Here's how the part is built. I have some questions about the finished solid (model axes, mm). A direction names the side the tool comes from. Coordinates: 2 decimals unless noted, no trailing zeros. Write each loop counter-clockwise with the first axis right and the second up, starting at its lowest first coordinate (ties: lowest second). Pieces come first, ordered by that corner, then holes.
(1) For pin 1 Ø5 at (x, y) = (5.75, -5.75) entering from -Z; pin 2 Ø4 at (x, y) = (-5.75, 5.75) entering from +Z, each with a flat end and sliding along its axis, tell me the tip position at first contact or that it passes through.
(2) Please list where these lines run through material, in increasing order: probe 1 along X at (y, z) = (5.75, 12.75); probe 2 along X at (y, z) = (-0.25, 14); probe 3 along X at (y, z) = (-5.75, 11.75).
(3) Which directions (+Z, -Z, +X, -X, +Y, -Y) give clear straight access to the entire face, cutting with the end or side of a thin tool? Please do faces 4 (the cylindrical face through (8.8, -2.36, 7.693)), 5 (the cylindrical face through (-14.292, 10.035, 11.352)), 6 (the cylindrical face through (6.49, 4.33, 9.68)), 7 (the flat face through (-8.7, 6, 2)), 8 (the cylindrical face through (5.97, 9.36, 17.29)).
(4) Imagine slicing it at A-A, the plane z = 10. List the corners of the cut face in (x, y) for me, plus the area to 3 significant figures.
(5) Imagine slicing it at C-C, the plane x = 0. List the corners of the cut face in (y, z) for me, plus the area to 3 significant figures.
(6) Imagine slicing it at D-D, the plane y = 1.25. List the corners of the cut face in (x, z) for me.
(7) Thinking about a two-plate mould opening in Z: for faces 1 (the cylindrical face through (-6.1, -7.31, 9.68)), 2 (the cylindrical face through (5.708, 10.035, 11.352)), 3 (the flat face through (6, 4, 5)), which applies, released by +Z, released by -Z, zero draft, split by the parting line, or undercut?
```python
from build123d import *

# Parameters (mm, degrees)
F0_W      = 40
F0_H      = 25
F0_R      = 1.6
F0_R_2    = 5.1
F1_DEPTH  = 20
F2_R      = 5
F3_R      = 11.1
F4_DEPTH  = 5.5
F5_R      = 1.6
F6_DEPTH  = 5
F7_R      = 2.6
F8_DEPTH  = 25.001
F9_R      = 4.5
F9_R_2    = 2.6
F10_DEPTH = 5


with BuildPart() as f1:
    # F0 (on Top) → F1 (new body)
    with BuildSketch(Plane.XY):
        Rectangle(F0_W, F0_H)
        with Locations((-5.75, -5.75)):
            Circle(F0_R, mode=Mode.SUBTRACT)
        with Locations((5.75, -5.75)):
            Circle(F0_R, mode=Mode.SUBTRACT)
        with Locations((-5.75, 5.75)):
            Circle(F0_R, mode=Mode.SUBTRACT)
        Circle(F0_R_2, mode=Mode.SUBTRACT)
        with Locations((5.75, 5.75)):
            Circle(F0_R, mode=Mode.SUBTRACT)
    extrude(amount=F1_DEPTH)

    # F2
    f2_edges = [f1.edges().sort_by_distance(p)[0] for p in [
        (20, 12.5, 10),
        (-20, 12.5, 10),
    ]]
    fillet(f2_edges, radius=F2_R)

    # F3 (on face) → F4 (cut)
    with BuildSketch(Plane.XY.offset(20)):
        Circle(F3_R)
    extrude(amount=-F4_DEPTH, mode=Mode.SUBTRACT)

    # F5 (on face) → F6 (cut)
    with BuildSketch(Plane(origin=(0, 0, 0), x_dir=(1, 0, 0), z_dir=(0, 0, -1))):
        Polygon((8.7, 7.423624), (5.735692, 8.977306), (2.8, 7.438623), (2.8, 4.076827), (5.75, 2.530645), (8.7, 4.076827), align=None)
        Polygon((8.7, -4.076376), (5.735692, -2.522694), (2.8, -4.061377), (2.8, -7.423173), (5.75, -8.969355), (8.7, -7.423173), align=None)
        with Locations((5.75, -5.75)):
            Circle(F5_R, mode=Mode.SUBTRACT)
        Polygon((-2.8, -4.076376), (-5.764308, -2.522694), (-8.7, -4.061377), (-8.7, -7.423173), (-5.75, -8.969355), (-2.8, -7.423173), align=None)
        with Locations((-5.75, -5.75)):
            Circle(F5_R, mode=Mode.SUBTRACT)
        Polygon((-2.8, 7.423624), (-5.764308, 8.977306), (-8.7, 7.438623), (-8.7, 4.076827), (-5.75, 2.530645), (-2.8, 4.076827), align=None)
        with Locations((-5.75, 5.75)):
            Circle(F5_R, mode=Mode.SUBTRACT)
    extrude(amount=-F6_DEPTH, mode=Mode.SUBTRACT)

    # F7 (on face) → F8 (cut, through all)
    with BuildSketch(Plane(origin=(0, 12.5, 0), x_dir=(-1, 0, 0), z_dir=(0, 1, 0))):
        with Locations((-10, 10)):
            Circle(F7_R)
        with Locations((10, 10)):
            Circle(F7_R)
    extrude(amount=-F8_DEPTH, mode=Mode.SUBTRACT)

    # F9 (on face) → F10 (cut)
    with BuildSketch(Plane(origin=(0, 12.5, 0), x_dir=(-1, 0, 0), z_dir=(0, 1, 0))):
        with Locations((10, 10)):
            Circle(F9_R)
        with Locations((10, 10)):
            Circle(F9_R_2, mode=Mode.SUBTRACT)
        with Locations((-10, 10)):
            Circle(F9_R)
        with Locations((-10, 10)):
            Circle(F9_R_2, mode=Mode.SUBTRACT)
    extrude(amount=-F10_DEPTH, mode=Mode.SUBTRACT)


solid = f1.part
```
Recorded:
1. pin 1: stops at z = 5
1. pin 2: stops at z = 14.5
2. probe 1: x = -20 to -7.35, -4.15 to 4.15, 7.35 to 20
2. probe 2: x = -20 to -5.09, 5.09 to 20
2. probe 3: x = -20 to -11.92, -8.08 to -7.35, -4.15 to 4.15, 7.35 to 8.08, 11.92 to 20
3. face 4: +Y, -Y
3. face 5: +Y
3. face 6: +Z, -Z
3. face 7: -Z
3. face 8: +Z
4. outline: (-20, -12.5) - (-12.6, -12.5) - (-12.6, 7.5) - (-14.5, 7.5) - (-14.5, 12.5) - (-15, 12.5) arc R5 ccw to (-20, 7.5) - close; (-7.4, -12.5) - (7.4, -12.5) - (7.4, 7.5) - (5.5, 7.5) - (5.5, 12.5) - (-5.5, 12.5) - (-5.5, 7.5) - (-7.4, 7.5) - close; (12.6, -12.5) - (20, -12.5) - (20, 7.5) arc R5 ccw to (15, 12.5) - (14.5, 12.5) - (14.5, 7.5) - (12.6, 7.5) - close; hole circle Ø3.2 at (-5.75, -5.75); hole circle Ø3.2 at (-5.75, 5.75); hole circle Ø10.2 at (0, 0); hole circle Ø3.2 at (5.75, -5.75); hole circle Ø3.2 at (5.75, 5.75)
4. area: 577 mm2
5. outline: (-12.5, 0) - (-5.1, 0) - (-5.1, 14.5) - (-11.1, 14.5) - (-11.1, 20) - (-12.5, 20) - close; (5.1, 0) - (12.5, 0) - (12.5, 20) - (11.1, 20) - (11.1, 14.5) - (5.1, 14.5) - close
5. area: 230 mm2
6. outline: (-20, 0) - (-4.94, 0) - (-4.94, 14.5) - (-11.03, 14.5) - (-11.03, 20) - (-20, 20) - close; (4.94, 0) - (20, 0) - (20, 20) - (11.03, 20) - (11.03, 14.5) - (4.94, 14.5) - close; hole circle Ø5.2 at (-10, 10); hole circle Ø5.2 at (10, 10)
7. face 1: zero draft
7. face 2: undercut
7. face 3: released by -Z
